Input: part model. Units: mm. Frame: model coordinates. Face numbers are marked on the shaded views. Coordinates: 2 decimals unless noted, no trailing zeros. Write each loop counter-clockwise with the first axis right and the second up, starting at its lowest first coordinate (ties: lowest second). Pieces come first, ordered by that corner, then holes. Notation, with made-up numbers: (84.5, 18.5) - (139.5, 18.5) arc R11 ccw to (139.5, 37.5) - close; hole circle Ø1 at (21, -36.75). An arc over 180 degrees is marked (long way). Use CSV: the item, a comma, the result in double quotes.
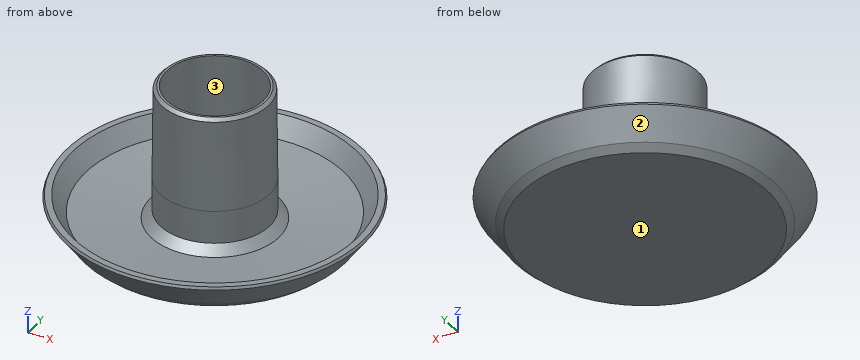
```python
from build123d import *

# Parameters (mm, degrees)
F2_SIZE  = 10
F3_SIZE  = 3
F4_SIZE2 = 0.3
F4_SIZE  = 30
F5_SIZE  = 1
F6_SIZE  = 1


with BuildPart() as f1:
    # F0 (on Front) → F1 (revolve)
    with BuildSketch(Plane.XZ):
        Polygon((15.35, 1.3613448423), (0, 0), (15.35, 0), align=None)
        Polygon((15.35, 0), (0, 0), (0, -2), (38.9759652317, -2), (41.235409677, 0), (35, 0), (17.35, 0), align=None)
        Polygon((15.35, 1.3613448423), (15.35, 0), (17.35, 0), (17.35, 1.5387187631), align=None)
        Polygon((15.35, 44.9680350721), (15.35, 1.3613448423), (17.35, 1.5387187631), (17.35, 44.9680350721), align=None)
        Polygon((17.35, 1.5387187631), (17.35, 0), (35, 0), (41.235409677, 0), (48, 9.3012940374), (45, 9.3012940374), (40.9695953131, 3.6334688775), align=None)
    revolve(axis=Axis((0, 0, 15.92751313), (0, 0, -1)))

    # F2
    f2_edges = [f1.edges().sort_by_distance(p)[0] for p in [
        (-15.35, 0, 1.361345),
    ]]
    chamfer(f2_edges, length=F2_SIZE)

    # F3
    f3_edges = [f1.edges().sort_by_distance(p)[0] for p in [
        (-17.35, 0, 1.538719),
    ]]
    chamfer(f3_edges, length=F3_SIZE)

    # F4
    f4_edges = [f1.edges().sort_by_distance(p)[0] for p in [
        (-17.35, 0, 44.968035),
    ]]
    f4_side = f1.faces().sort_by_distance((-17.35, 0, 24.753377))[0]
    chamfer(f4_edges, length=F4_SIZE, length2=F4_SIZE2, reference=f4_side)

    # F5
    f5_edges = [f1.edges().sort_by_distance(p)[0] for p in [
        (-48, 0, 9.301294),
    ]]
    chamfer(f5_edges, length=F5_SIZE)

    # F6
    f6_edges = [f1.edges().sort_by_distance(p)[0] for p in [
        (-17.05, 0, 44.968035),
    ]]
    chamfer(f6_edges, length=F6_SIZE)


solid = f1.part
```
(1) Pin query (flat end, axial travel): pin 1 Ø1 at (y, z) = (12.5, 17) entering from +X; pin 2 Ø10 at (x, z) = (-15.5, 40) entering from -Y; pin 3 Ø3 at (x, z) = (10, 34.5) entering from +Y. Return the tip coordinate at first contact, or that it passes through.
Check values:
pin 1,"x = 12.5"
pin 2,"y = -13.5"
pin 3,"y = 14.9"
(2) Ray query, probe 1 along X at (y, z) = (0, 21.5); probe 2 along Y at (x, z) = (0, 19); probe 3 along X at (y, z) = (-8.5, 33). Return the intervals inside material, ascending. Write a range as from..to.
Check values:
probe 1,"-17.28..-15.35, 15.35..17.28"
probe 2,"-17.31..-15.35, 15.35..17.31"
probe 3,"-14.92..-12.78, 12.78..14.92"
(3) Draft query along Y for the marked faces 1, 2 and 3. Return one class per face: pulls with the +Y half, pulls with the -Y half, needs draft (parallel to the pull), parting line crosses it, or undercut.
Check values:
face 1,"needs draft"
face 2,"parting line crosses it"
face 3,"undercut"
(4) Cut plane A-A on z = 18. Return loops of the section in (x, y), and give its area (3 significant figures).
Check values:
outline,"circle Ø34.64 at (0, 0); hole circle Ø30.7 at (0, 0)"
area,"202 mm^2"
